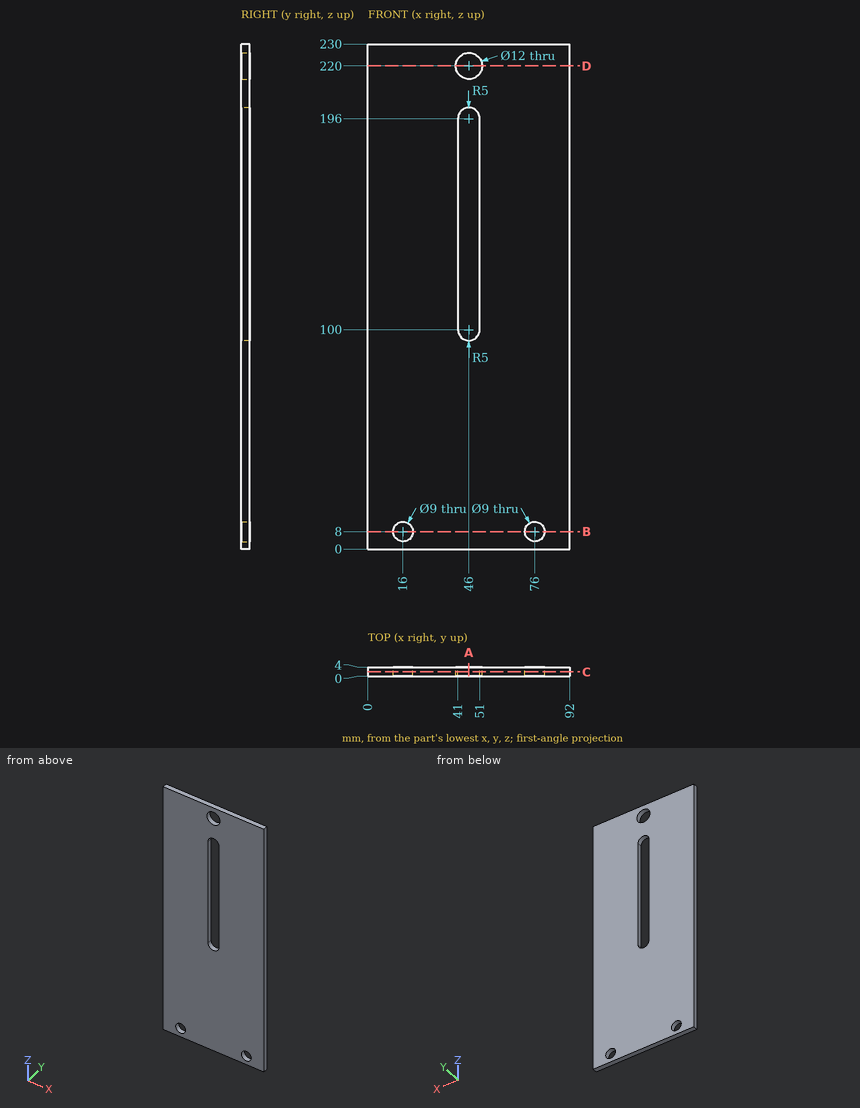
Job drawing, mm, ordinate dimensions from the low corner. One solid piece. Coordinates: 2 decimals unless noted, no trailing zeros. Order: outer loops, then holes, each group sorted by start corner. A loop starts at its lowest first (then second) coordinate and runs counter-clockwise, first axis right, second up. Notation, with made-up numbers: (-7, -21.5) -> (38, -21.5) arc R30 ccw to (38, 0.5) -> close; hole circle Ø3 at (25.5, 62). An arc over 180 degrees is marked (long way). Return JSON: item names as keys, results as strings. Group by question number.
Item 1: Saw through at C-C on y = 1.85. Write the cut outline in (x, z).
Item 2: Saw through at D-D on z = 220. Write the cut outline in (x, y).
Item 3: Wall check: line 1 along Z through (x, y) = (46, 2.1); line 2 along Z through (x, y) = (76, 2.45); line 3 along X through (y, z) = (3.4, 127.5). Give the ranges that are in metal, low to high. Write a range as [from, to].
Item 4: Saw through at A-A on x = 46. Write the cut outline in (y, z), then the cut area to 3 significant figures.
Item 5: Saw through at B-B on z = 8. Write the cut outline in (x, y), then the cut area to 3 significant figures.
Values found:
{
 "1": {"outline": "(0, 0) -> (92, 0) -> (92, 230) -> (0, 230) -> close; hole circle Ø9 at (16, 8); hole circle Ø12 at (46, 220); hole (41, 100) arc R5 ccw to (51, 100) -> (51, 196) arc R5 ccw to (41, 196) -> close; hole circle Ø9 at (76, 8)"},
 "2": {"outline": "(0, 0) -> (40, 0) -> (40, 4) -> (0, 4) -> close; (52, 0) -> (92, 0) -> (92, 4) -> (52, 4) -> close"},
 "3": {"line 1": "z = [0, 95], [201, 214], [226, 230]", "line 2": "z = [0, 3.5], [12.5, 230]", "line 3": "x = [0, 41], [51, 92]"},
 "4": {"outline": "(0, 0) -> (4, 0) -> (4, 95) -> (0, 95) -> close; (0, 201) -> (4, 201) -> (4, 214) -> (0, 214) -> close; (0, 226) -> (4, 226) -> (4, 230) -> (0, 230) -> close", "area": "448 mm2"},
 "5": {"outline": "(0, 0) -> (11.5, 0) -> (11.5, 4) -> (0, 4) -> close; (20.5, 0) -> (71.5, 0) -> (71.5, 4) -> (20.5, 4) -> close; (80.5, 0) -> (92, 0) -> (92, 4) -> (80.5, 4) -> close", "area": "296 mm2"}
}
